```python
from build123d import *

# Parameters (mm, degrees)
BOSS_EXTRUDE1_DEPTH = 2.794
SKETCH2_W           = 6.35
SKETCH2_H           = 5.588
BOSS_EXTRUDE2_DEPTH = 2.794
SKETCH4_R           = 11.1125
CUT_EXTRUDE2_DEPTH  = 35.803228508
FILLET1_R           = 2.54


with BuildPart() as part:
    # Sketch1 → Boss-Extrude1 (new, symmetric)
    with BuildSketch(Plane(origin=(0, 0, 0), x_dir=(1, 0, 0), z_dir=(0, 1, 0))):
        Polygon((-13.81125, 22.225), (-19.52625, 22.225), (-19.52625, -3.27025), (-16.47825, -6.31825), (-13.93825, -6.31825), (-13.93825, -11.90625), (-16.47825, -11.90625), (-19.52625, -14.95425), (-19.52625, -22.225), (-13.81125, -22.225), (-6.82625, -22.225), (-6.82625, -27.813), (13.81125, -27.813), (13.81125, -22.225), (13.81125, 22.225), (13.81125, 27.813), (-6.82625, 27.813), (-6.82625, 22.225), align=None)
    extrude(amount=BOSS_EXTRUDE1_DEPTH, both=True)

    # Sketch2 → Boss-Extrude2 (add, symmetric)
    with BuildSketch(Plane(origin=(0, 0, 0), x_dir=(1, 0, 0), z_dir=(0, 1, 0))):
        with Locations((16.98625, 0)):
            Rectangle(SKETCH2_W, SKETCH2_H)
    extrude(amount=BOSS_EXTRUDE2_DEPTH, both=True)

    # Sketch4 → Cut-Extrude2 (cut, through all)
    with BuildSketch(Plane(origin=(0, 2.794, 0), x_dir=(1, 0, 0), z_dir=(0, 1, 0))):
        with Locations(Location((-0.604747552, 0, 0), (0, 0, 270))):
            Circle(SKETCH4_R)
    extrude(amount=-CUT_EXTRUDE2_DEPTH, mode=Mode.SUBTRACT)

    # Fillet1
    fillet1_edges = [part.edges().sort_by_distance(p)[0] for p in [
        (-19.52625, 0, 22.225),
        (-19.52625, 0, -22.225),
    ]]
    fillet(fillet1_edges, radius=FILLET1_R)


solid = part.part
```
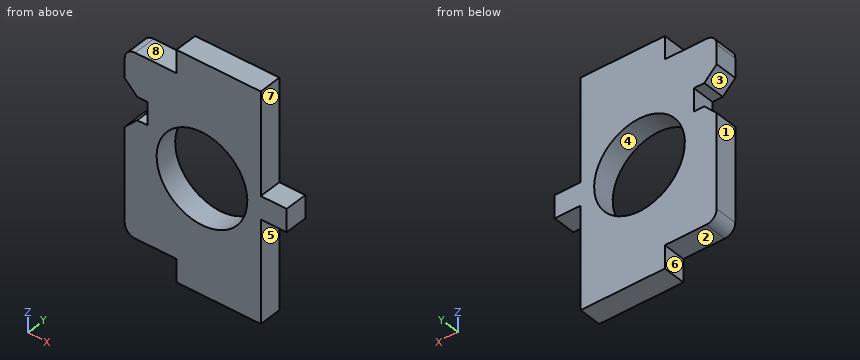
Check sheet for the modelled part. Datum: model origin and axes. Units: mm. Face numbers are marked on the shaded views. A direction names the side the tool comes from. Round coordinates to 2 decimals unless told otherwise and drop trailing zeros. Order: outer loops, then holes, each group sorted by start corner. A loop starts at its lowest first (then second) coordinate and runs counter-clockwise, first axis right, second up. Notation, with made-up numbers: (67.25, -18) -> (81.25, -18) arc R24 cw to (81.25, 5) -> close; hole circle Ø4 at (-30.75, 31). An arc over 180 degrees is marked (long way). One line per item, written item: value. Start each with the question number.
Q1. Cross-section at C-C (y = -0.7). Record the boundary of the cut face in (x, z) (1 decimal), and give its area (3 significant figures).
Q2. Set-up check for the marked faces 5, 6, 7 and 8: record each of +Z, -Z, +X, -X, +Y, -Y from which the full face is reachable in a straight line by a thin tool's end or side.
Q3. Cross-section at A-A (x = -14.5). Record the boundary of the cut face in (y, z) (3 decimals), and give its area (3 significant figures).
Q4. Cross-section at D-D (z = 16). Record the boundary of the cut face in (x, y), and give its area (3 significant figures).
Q5. Gauge pin test, flat ends, axial feed: pin 1 Ø1.7 at (x, y) = (16, -1.5) entering from -Z; pin 2 Ø1.7 at (y, z) = (-1.5, -14) entering from +X; pin 3 Ø1.7 at (x, y) = (-14, -0.5) entering from +Z (3 decimals); pin 4 Ø8 at (x, z) = (-10, 4.5) entering from -Y. Record the tip position at first contact, or that the pin passes through.
Q6. Cross-section at B-B (z = 0). Record the boundary of the cut face in (x, y).
Q7. Mould release check, pull along Z, two halves, no side actions. Record for the marked faces 1, 2, 3 and 4: pulls with the +Z half, pulls with the -Z half, needs draft (parallel to the pull), parting line crosses it, or undercut.
Q8. Thickness scan on line 1 (X direction, y = -0.45, z = 0); line 2 (Z direction, x = 18, y = -0.85); line 3 (X direction, y = -1.7, z = 15). Record the ranges inside material, lowest first.
Completed:
1. outline: (-19.5, -19.7) arc R2.5 ccw to (-17, -22.2) -> (-6.8, -22.2) -> (-6.8, -27.8) -> (13.8, -27.8) -> (13.8, -2.8) -> (20.2, -2.8) -> (20.2, 2.8) -> (13.8, 2.8) -> (13.8, 27.8) -> (-6.8, 27.8) -> (-6.8, 22.2) -> (-17, 22.2) arc R2.5 ccw to (-19.5, 19.7) -> (-19.5, 15) -> (-16.5, 11.9) -> (-13.9, 11.9) -> (-13.9, 6.3) -> (-16.5, 6.3) -> (-19.5, 3.3) -> close; hole circle Ø22.2 at (-0.6, 0)
1. area: 1,320 mm²
2. face 5: -Z, +X, +Y, -Y
2. face 6: -Z, -X, +Y, -Y
2. face 7: +Z, +X, +Y, -Y
2. face 8: +Z, -X, +Y, -Y
3. outline: (-2.794, -22.225) -> (2.794, -22.225) -> (2.794, 6.318) -> (-2.794, 6.318) -> close; (-2.794, 11.906) -> (2.794, 11.906) -> (2.794, 22.225) -> (-2.794, 22.225) -> close
3. area: 217 mm²
4. outline: (-19.53, -2.79) -> (13.81, -2.79) -> (13.81, 2.79) -> (-19.53, 2.79) -> close
4. area: 186 mm²
5. pin 1: stops at z = -2.79
5. pin 2: stops at x = 13.81
5. pin 3: stops at z = 22.225
5. pin 4: stops at y = -2.79
6. outline: (-19.53, -2.79) -> (-11.72, -2.79) -> (-11.72, 2.79) -> (-19.53, 2.79) -> close; (10.51, -2.79) -> (20.16, -2.79) -> (20.16, 2.79) -> (10.51, 2.79) -> close
7. face 1: needs draft
7. face 2: pulls with the -Z half
7. face 3: undercut
7. face 4: undercut
8. line 1: x = -19.53 to -11.72, 10.51 to 20.16
8. line 2: z = -2.79 to 2.79
8. line 3: x = -19.53 to 13.81
